from build123d import *

# Parameters (mm, degrees)
PAD_DEPTH    = 5
SKETCH002_R  = 9.228742
PAD001_DEPTH = 25
POCKET_DEPTH = 25


with BuildPart() as part:
    # Sketch001 → Pad (new body)
    with BuildSketch(Plane.XY):
        Polygon((0, 10), (80, 10), (80, 50), (100, 50), (100, -50), (80, -50), (80, -10), (0, -10), (-80, -10), (-80, -50), (-100, -50), (-100, 50), (-80, 50), (-80, 10), align=None)
    extrude(amount=PAD_DEPTH)

    # Sketch002 → Pad001 (new body)
    with BuildSketch(Plane.XY.offset(5)):
        with Locations((90, 0)):
            Circle(SKETCH002_R)
        with Locations((-90, 0)):
            Circle(SKETCH002_R)
    extrude(amount=PAD001_DEPTH)

    # Sketch003 → Pocket (cut)
    with BuildSketch(Plane.XY.offset(30)):
        Polygon((-87.480573, 3.871152), (-92.092803, 4.117464), (-94.61223, 0.246312), (-92.519427, -3.871152), (-87.907197, -4.117464), (-85.38777, -0.246312), align=None)
    pocket = extrude(amount=-POCKET_DEPTH, mode=Mode.SUBTRACT)

    # Mirrored: Pocket across Sketch003 V_Axis
    add(pocket.mirror(Plane(origin=(0, 0, 30), x_dir=(0, 0, 1), z_dir=(1, 0, 0))), mode=Mode.SUBTRACT)


solid = part.part
Read the model definition and answer for the solid it produces. Units are mm, in the model's axes. A direction names the side the tool comes from. Give positions to 0.01 mm unless a question says otherwise; leave off trailing zeros. Write each loop counter-clockwise with the first axis right and the second up, starting at its lowest first coordinate (ties: lowest second). Pieces come first, ordered by that corner, then holes. Notation, with made-up numbers: (5, 73) - (44, 73) arc R15 ccw to (44, 95) - close; hole circle Ø1 at (79.25, 64.5). An arc over 180 degrees is marked (long way). Return JSON: item names as keys, results as strings.
Q1. A cutting plane is placed at C-C, the plane x = -90. Determine the outline of the cut face in (y, z).
Reply:
{"outline": "(-50, 0) - (50, 0) - (50, 5) - (9.23, 5) - (9.23, 30) - (4.01, 30) - (4.01, 5) - (-4.01, 5) - (-4.01, 30) - (-9.23, 30) - (-9.23, 5) - (-50, 5) - close"}
Q2. A cutting plane is placed at A-A, the plane z = 12.25. Determine the outline of the cut face in (x, y).
Reply:
{"outline": "circle Ø18.46 at (-90, 0); circle Ø18.46 at (90, 0); hole (-94.61, 0.25) - (-92.52, -3.87) - (-87.91, -4.12) - (-85.39, -0.25) - (-87.48, 3.87) - (-92.09, 4.12) - close; hole (85.39, -0.25) - (87.91, -4.12) - (92.52, -3.87) - (94.61, 0.25) - (92.09, 4.12) - (87.48, 3.87) - close"}
Q3. For faces 1 (the face through (-1, -10, 2)), 2 (the face through (-80, 30, 2)), 3 (the face through (-93.58, -1.784, 17.675)), determine the directions among +Z, -Z, +X, -X, +Y, -Y from which every point of the face is accessible in a straight line to the end or side of a thin tool.
Reply:
{"face 1": "+Z, -Z, -Y", "face 2": "+Z, -Z, +Y", "face 3": "+Z"}
Q4. A cutting plane is placed at B-B, the plane y = 17. Determine the outline of the cut face in (x, z).
Reply:
{"outline": "(-100, 0) - (-80, 0) - (-80, 5) - (-100, 5) - close; (80, 0) - (100, 0) - (100, 5) - (80, 5) - close"}
Q5. Consider line 1 along X through (y, z) = (-40.5, 4.5); line 2 along X through (y, z) = (-2.5, 22.25); line 3 along X through (y, z) = (-3, 10.5). Determine where each line is inside the solid, lowest interval first. Write a range as [from, to].
Reply:
{"line 1": "[-100, -80], [80, 100]", "line 2": "[-98.88, -93.22], [-86.85, -81.12], [81.12, 86.85], [93.22, 98.88]", "line 3": "[-98.73, -92.96], [-87.18, -81.27], [81.27, 87.18], [92.96, 98.73]"}
Q6. A cutting plane is placed at D-D, the plane x = -49. Determine the outline of the cut face in (y, z), and give its area (3 significant figures).
Reply:
{"outline": "(-10, 0) - (10, 0) - (10, 5) - (-10, 5) - close", "area": "100 mm²"}
Q7. For a pull along X with two mould halves and no side action, classify faces 4 (the face through (90, 50, 2)), 5 (the face through (80, 30, 2)), 6 (the face through (100, 1, 2)), 7 (the face through (80, -30, 2)) as released by +X, released by -X, zero draft, split by the parting line, or undercut.
Reply:
{"face 4": "zero draft", "face 5": "undercut", "face 6": "released by +X", "face 7": "undercut"}
Q8. Given P1, Ø6.5, axis at x = 90, y = 0.5, coming from the +Z side; P2, Ø1, axis at y = 11.5, z = 26, coming from the +X side; P3, Ø5, axis at y = -9.5, z = 23.5, coming from the -X side; P4, Ø4, axis at x = 17.5, z = 2.5, coming from the +Y side, each flat-ended and moving along its own axis, determine where each tip first touches the part or whether it passes through.
Reply:
{"P1": "z = 5", "P2": "through", "P3": "x = -96.01", "P4": "y = 10"}
